Verification items for this drawing (mm, ordinates from the low corner). Round coordinates to 2 decimals unless told otherwise and drop trailing zeros. Write each loop counter-clockwise with the first axis right and the second up, starting at its lowest first coordinate (ties: lowest second). Pieces come first, ordered by that corner, then holes.
Item 1: Draft check along Z on the marked faces 1, 2 and 3. Enter one of: pulls with the +Z half, pulls with the -Z half, needs draft (parallel to the pull), parting line crosses it, or undercut.
Item 2: Depth check by flat-ended pin: P1, Ø4, axis at y = 192, z = 104, coming from the -X side (1 decimal); P2, Ø3, axis at x = 412, y = 36, coming from the +Z side; P3, Ø2, axis at y = 150, z = 40, coming from the -X side; P4, Ø4, axis at y = 49.5, z = 106, coming from the -X side. Enter the tip coordinate at first touch or a pass-through.
Item 3: Cross-section at B-B (x = 453.5). Enter the section's corners in (y, z) (1 decimal).
Item 4: Cross-section at A-A (y = 185.5). Enter the section's corners in (x, z), then the cut area to 3 significant figures.
Item 5: Scan lines: probe 1 along Z at (x, y) = (42.5, 19); probe 2 along Z at (x, y) = (456.5, 32); probe 3 along X at (y, z) = (183, 105). Record each from-to range of solid material in increasing order.
Item 6: Cross-section at C-C (z = 100). Enter the section's corners in (x, y) (1 decimal).
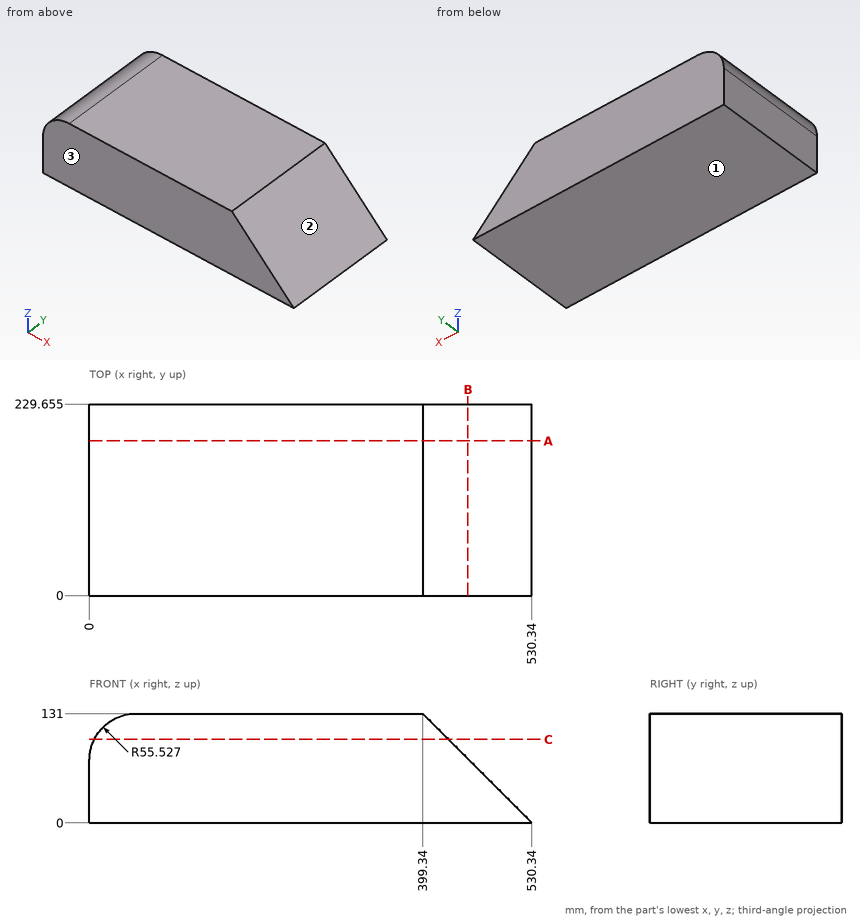
Resolved:
1. face 1: pulls with the -Z half
1. face 2: pulls with the +Z half
1. face 3: needs draft
2. P1: stops at x = 6.7
2. P2: stops at z = 119.84
2. P3: stops at x = 0
2. P4: stops at x = 7.89
3. outline: (0, 0) - (229.7, 0) - (229.7, 76.8) - (0, 76.8) - close
4. outline: (0, 0) - (530.34, 0) - (399.34, 131) - (55.53, 131) arc R55.53 ccw to (0, 75.47) - close
4. area: 60,200 mm2
5. probe 1: z = 0 to 129.45
5. probe 2: z = 0 to 73.84
5. probe 3: x = 8.5 to 425.34
6. outline: (5.7, 0) - (430.3, 0) - (430.3, 229.7) - (5.7, 229.7) - close
